Part model, mm, in its own coordinate system. Face numbers are marked on the shaded views. A direction names the side the tool comes from. Coordinates: 2 decimals unless noted, no trailing zeros. Write each loop counter-clockwise with the first axis right and the second up, starting at its lowest first coordinate (ties: lowest second). Pieces come first, ordered by that corner, then holes. Notation, with made-up numbers: (-15.5, 83) -> (8.5, 83) arc R34 ccw to (8.5, 114) -> close; hole circle Ø11 at (82, 54). An arc over 180 degrees is marked (long way). One line per question, with ' | ' between items. Start each with the question number.
Item 1: Saw through at A-A (y = 0). List the corners of the cut face in (x, z), and give its area (3 significant figures).
Item 2: Saw through at B-B (z = -2.5). List the corners of the cut face in (x, y).
Item 3: Saw through at C-C (x = 0). List the corners of the cut face in (y, z), and give its area (3 significant figures).
Item 4: Probe probe 1 along Y at (x, z) = (0, 0.1); probe 2 along Y at (x, z) = (0, -2.6); probe 3 along Z at (x, y) = (-1.5, 2.75). List the from-to ranges inside material, lowest first. Write a range as [from, to].
Item 5: Pin check, flat tips, straight feed: pin 1 (0.6 mm diameter, centred on y = -2, z = -3, fed in from +X); pin 2 (0.8 mm diameter, centred on x = 1.5, y = 0.5, fed in from -Z). Stop position of each tip, or through.
Item 6: 3-axis set-ups, long thin cutter, end or side, ignore diameter. For the marked faces 1, 2 and 3: which of +Z, -Z, +X, -X, +Y, -Y reach the whole face in a straight line?
Item 7: Saw through at D-D (z = -1.5). List the corners of the cut face in (x, y).
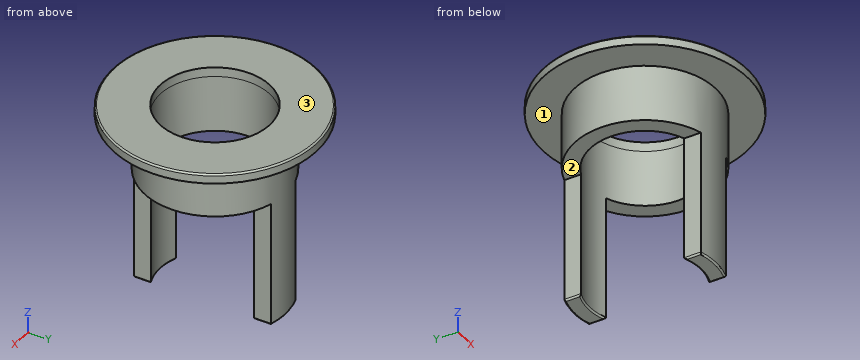
from build123d import *

# Parameters (mm, degrees)
SKETCH_1_R          = 3.25
SKETCH_1_R_2        = 2.25
SKETCH_1_R_3        = 1.75
EXTRUDE_1_DEPTH     = 0.3
SKETCH_1_4_R        = 2.25
SKETCH_1_4_R_2      = 1.75
EXTRUDE_2_DEPTH     = 5.8
CUT_EXTRUDE_1_DEPTH = 4
FILLET_1_R          = 0.05


with BuildPart() as part:
    # Sketch 1 → Extrude 1 (new body)
    with BuildSketch(Plane.XY):
        Circle(SKETCH_1_R)
        Circle(SKETCH_1_R_2, mode=Mode.SUBTRACT)
        Circle(SKETCH_1_R_2)
        Circle(SKETCH_1_R_3, mode=Mode.SUBTRACT)
    extrude(amount=EXTRUDE_1_DEPTH)

    # Sketch 1_4 → Extrude 2 (add)
    with BuildSketch(Plane.XY):
        Circle(SKETCH_1_4_R)
        Circle(SKETCH_1_4_R_2, mode=Mode.SUBTRACT)
    extrude(amount=-EXTRUDE_2_DEPTH)

    # Sketch 2 → Cut-Extrude 1 (cut)
    with BuildSketch(Plane(origin=(0, 0, -5.8), x_dir=(-1, 0, 0), z_dir=(0, 0, -1))):
        with BuildLine():
            ThreePointArc((-0.65, 2.154065923), (-2.25, 0), (-0.65, -2.154065923))
            Line((-0.65, -2.154065923), (-0.65, -1.624807681))
            ThreePointArc((-0.65, -1.624807681), (-1.75, 0), (-0.65, 1.624807681))
            Line((-0.65, 1.624807681), (-0.65, 2.154065923))
        make_face()
        with BuildLine():
            Line((0.65, -1.624807681), (0.65, -2.154065923))
            ThreePointArc((0.65, -2.154065923), (1.806239187, -1.341640786), (2.25, 0))
            ThreePointArc((2.25, 0), (1.806239187, 1.341640786), (0.65, 2.154065923))
            Line((0.65, 2.154065923), (0.65, 1.624807681))
            ThreePointArc((0.65, 1.624807681), (1.449137675, 0.981070844), (1.75, 0))
            ThreePointArc((1.75, 0), (1.449137675, -0.981070844), (0.65, -1.624807681))
        make_face()
    extrude(amount=-CUT_EXTRUDE_1_DEPTH, mode=Mode.SUBTRACT)

    # Fillet 1
    fillet_1_edges = [part.edges().sort_by_distance(p)[0] for p in [
        (0, 1.75, -5.8),
        (0.65, -1.889436802, -5.8),
        (0.65, 1.889436802, -5.8),
        (0, -1.75, -5.8),
        (0, -2.25, -5.8),
        (-0.65, 1.889436802, -5.8),
        (-0.65, -1.889436802, -5.8),
        (-3.25, 0, 0.3),
        (0, 2.25, -5.8),
    ]]
    fillet(fillet_1_edges, radius=FILLET_1_R)


solid = part.part
From the geometry:
1) outline: (-3.25, 0) -> (-2.25, 0) -> (-2.25, -1.8) -> (-1.75, -1.8) -> (-1.75, 0.3) -> (-3.2, 0.3) arc R0.05 ccw to (-3.25, 0.25) -> close; (1.75, -1.8) -> (2.25, -1.8) -> (2.25, 0) -> (3.25, 0) -> (3.25, 0.25) arc R0.05 ccw to (3.2, 0.3) -> (1.75, 0.3) -> close | area: 2.70 mm2
2) outline: (-0.65, -2.15) arc R2.25 ccw to (0.65, -2.15) -> (0.65, -1.62) arc R1.75 cw to (-0.65, -1.62) -> close; (-0.65, 1.62) arc R1.75 cw to (0.65, 1.62) -> (0.65, 2.15) arc R2.25 ccw to (-0.65, 2.15) -> close
3) outline: (-3.25, 0) -> (-2.25, 0) -> (-2.25, -5.75) arc R0.05 ccw to (-2.2, -5.8) -> (-1.8, -5.8) arc R0.05 ccw to (-1.75, -5.75) -> (-1.75, 0.3) -> (-3.2, 0.3) arc R0.05 ccw to (-3.25, 0.25) -> close; (1.75, -5.75) arc R0.05 ccw to (1.8, -5.8) -> (2.2, -5.8) arc R0.05 ccw to (2.25, -5.75) -> (2.25, 0) -> (3.25, 0) -> (3.25, 0.25) arc R0.05 ccw to (3.2, 0.3) -> (1.75, 0.3) -> close | area: 6.70 mm2
4) probe 1: [-3.25, -1.75], [1.75, 3.25] | probe 2: [-2.25, -1.75], [1.75, 2.25] | probe 3: [0, 0.3]
5) pin 1: x = 0.65 | pin 2: z = -1.8
6) face 1: -Z | face 2: -Z, -X, +Y, -Y | face 3: +Z, +X, -X, +Y, -Y
7) outline: circle Ø4.5 at (0, 0); hole circle Ø3.5 at (0, 0)
